Study the drawing (mm; zero at the part's minimum x, y, z) and answer. Give positions to 0.01 mm unless a question says otherwise; leave off trailing zeros. Write each loop counter-clockwise with the first axis right and the second up, starting at its lowest first coordinate (ties: lowest second). Pieces come first, ordered by that corner, then holes. Notation, with made-up numbers: (9, 56.25) - (32, 56.25) arc R11 ccw to (32, 65.25) - close; hole circle Ø6 at (-14, 56). An arc over 180 degrees is marked (long way). Answer as CSV lines item,"result".
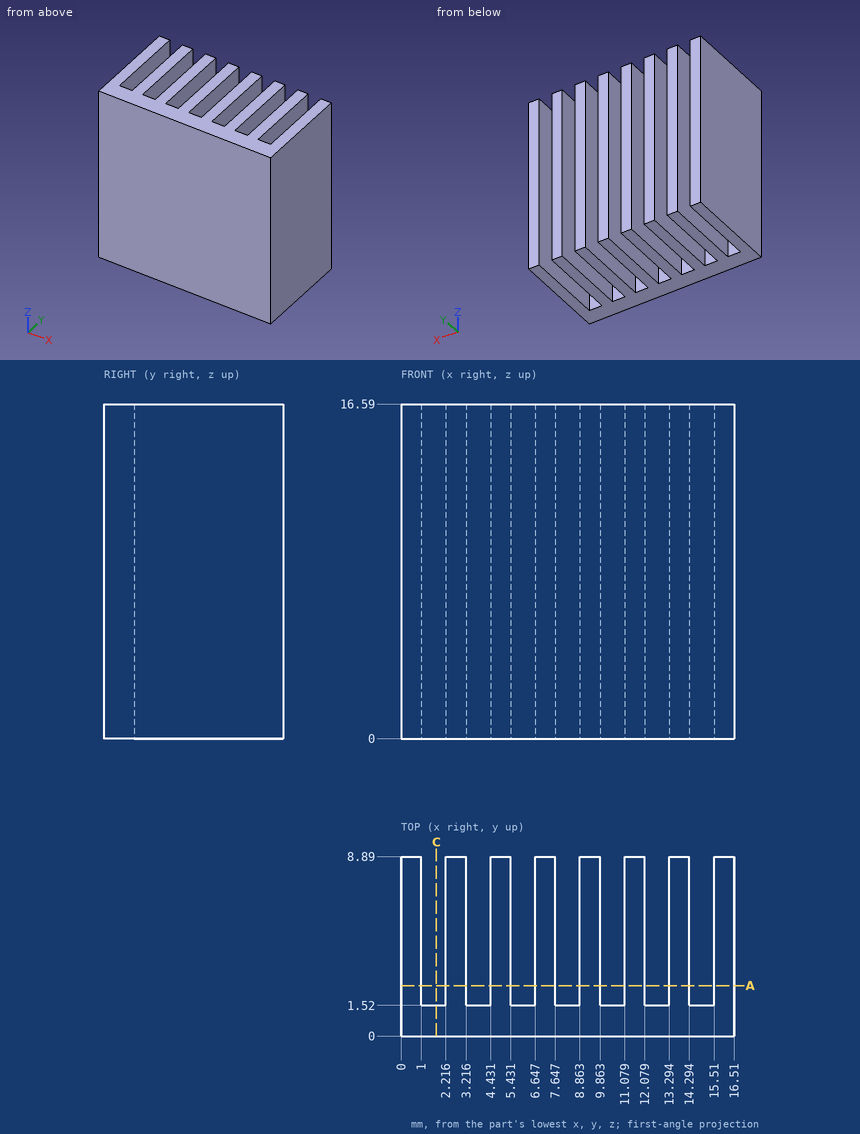
(1) A cutting plane is placed at C-C (x = 1.75). Write down the section's boundary in (y, z).
Worked out:
outline,"(0, 0) - (1.52, 0) - (1.52, 16.59) - (0, 16.59) - close"
(2) A cutting plane is placed at A-A (y = 2.5). Count the separate pieces of the cut face and the enclosed holes in it.
Worked out:
separate pieces,"8"
enclosed holes,"0"
(3) This flat-tipped pin is pushed along its axis until it touches: P1, Ø1, axis at x = 10.5, z = 8.5, coming from the +Y side. Where does it stop, or does it pass through?
Worked out:
P1,"stops at y = 1.52"
(4) Find the intervals of material crossed by L1, parallel to Y at x = 5.75, z = 2.5, in increasing order.
Worked out:
L1,"y = 0 to 1.52"
